```python
from build123d import *

# Parameters (mm, degrees)
F1_DEPTH    = 13.64111
F2_T1_DEPTH = 137.0825914491
F3_R        = 5.08
F4_SIZE     = 5.08
F5_R        = 5.08


# Not quite as in the source:
# - a fillet or chamfer that OpenCascade refuses, or shapes differently, is made with other operations: its cross-section is extruded or revolved along the edge and cut away or added


with BuildPart() as f1:
    # F0 (on Front) → F1 (new body)
    with BuildSketch(Plane.XZ):
        Polygon((0, 0), (16.8357715011, 14.2703205347), (38.0007438362, -20.6839479506), (71.29599154, 42.4681007862), (46.0088496082, 71.3043088503), (32.1346404756, 59.1376919794), (-23.249398917, 59.1376919794), (-38.0007401109, 41.5282361209), (-12.0255500078, 8.1773754209), (-43.7860488892, -80.4887861013), (-32.4603319168, -80.8862298727), align=None)
        Polygon((-32.4603319168, -214.6375030279), (-32.4603319168, -80.8862298727), (-43.7860488892, -80.4887861013), (-43.7860488892, -214.6375030279), align=None)
    extrude(amount=F1_DEPTH)

    # F2: chamfer of 7.62 x 12.7 on 2 edges, made by hand

    # F2_s2 → F2_t1 (cut)
    with BuildSketch(Plane(origin=(-15.5861012637, 0, -29.5626041102), x_dir=(0, 1, 0), z_dir=(0.4663751275, 0, 0.8845870451))):
        Polygon((-6.02111, -43.2614445663), (-13.64111, -30.5614445663), (-13.64111, -43.2614445663), align=None)
        Polygon((-7.62, -43.2614445663), (0, -30.5614445663), (0, -43.2614445663), align=None)
    extrude(amount=F2_T1_DEPTH, mode=Mode.SUBTRACT)

    # F3
    f3_edges = [f1.edges().sort_by_distance(p)[0] for p in [
        (-32.460332, -13.64111, -147.761866),
        (-32.460332, 0, -147.761866),
        (-43.786049, -13.64111, -147.563145),
        (-43.786049, 0, -147.563145),
        (-16.230166, -13.64111, -40.443115),
        (-27.905799, -13.64111, -36.155705),
        (-27.905799, 0, -36.155705),
        (-16.230166, 0, -40.443115),
    ]]
    fillet(f3_edges, radius=F3_R)

    # F4
    f4_edges = [f1.edges().sort_by_distance(p)[0] for p in [
        (39.071745, -13.64111, 65.221),
        (39.071745, 0, 65.221),
    ]]
    chamfer(f4_edges, length=F4_SIZE)

    # F5
    f5_edges = [f1.edges().sort_by_distance(p)[0] for p in [
        (-30.62507, -13.64111, 50.332964),
        (-30.62507, 0, 50.332964),
        (-25.013145, 0, 24.852806),
        (-25.013145, -13.64111, 24.852806),
        (4.442621, -13.64111, 59.137692),
        (4.442621, 0, 59.137692),
    ]]
    fillet(f5_edges, radius=F5_R)


solid = f1.part
```
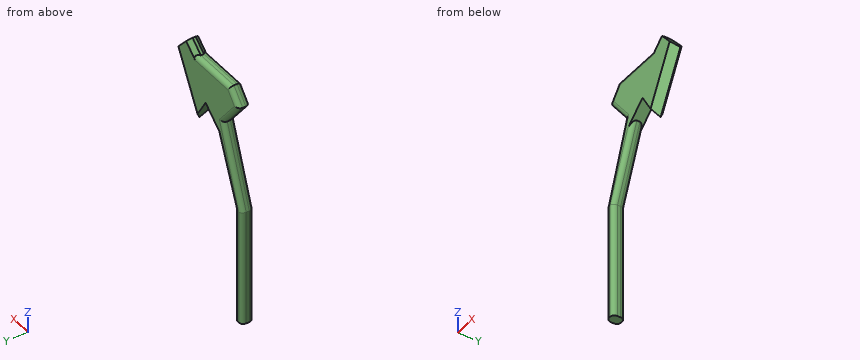
Input: part model. Units: mm. Frame: model coordinates. Give positions to 0.01 mm unless a question says otherwise; leave off trailing zeros. Order: outer loops, then holes, each group sorted by start corner. A loop starts at its lowest first (then second) coordinate and runs counter-clockwise, first axis right, second up.
1. Pin query (flat end, axial travel): pin 1 Ø2 at (x, y) = (24.5, -1.5) entering from -Z; pin 2 Ø1 at (x, y) = (34, -2) entering from +Z; pin 3 Ø8 at (x, y) = (-17.5, -8.5) entering from +Z. Return the tip coordinate at first contact, or that it passes through.
Computed:
pin 1: stops at z = -0.04
pin 2: stops at z = 58.43
pin 3: stops at z = 59.14
2. Cut plane A-A (z = -170). Return loops of the section in (x, y), and give its area (3 significant figures).
Computed:
outline: (-43.79, -8.56) arc R5.08 ccw to (-38.71, -13.64) - (-37.54, -13.64) arc R5.08 ccw to (-32.46, -8.56) - (-32.46, -5.08) arc R5.08 ccw to (-37.54, 0) - (-38.71, 0) arc R5.08 ccw to (-43.79, -5.08) - close
area: 132 mm2
3. Line query: probe 1 along X at (y, z) = (-6, 5); probe 2 along X at (y, z) = (-12.75, 6); probe 3 along X at (y, z) = (-7, -160.5). Output: solid intervals per line, ascending.
Computed:
probe 1: x = -13.16 to 5.9, 22.45 to 48.49
probe 2: x = -10.46 to 7.08, 21.84 to 39.39
probe 3: x = -43.79 to -32.46
4. Cut plane B-B (y = -2.5). Return loops of the section in (x, z), and give its area (3 significant figures).
Computed:
outline: (-43.08, -214.64) - (-33.16, -214.64) - (-33.16, -80.75) - (-1.15, -0.97) - (16.84, 14.27) - (32.84, -12.17) - (65.27, 49.34) - (47.71, 69.36) - (35.25, 58.43) - (-22.92, 58.43) - (-37.1, 41.51) - (-11.23, 8.3) - (-43.08, -80.61) - close
area: 6,850 mm2
